from build123d import *

# Parameters (mm, degrees)
SALIENTE_EXTRUIR1_DEPTH    = 4.91
VACIADO1_T                 = -1.95
CROQUIS3_R                 = 2
SALIENTE_EXTRUIR3_DEPTH    = 2.96
CORTAR_EXTRUIR1_DEPTH      = 68.872038609
CORTAR_EXTRUIR1_DEPTH_BACK = 2.96
CROQUIS4_R                 = 1


with BuildPart() as part:
    # Croquis1 → Saliente-Extruir1 (new body)
    with BuildSketch(Plane.XY):
        Polygon((-54.055, -12.97), (-54.055, -40.75), (54.055, -40.75), (54.055, -12.97), (48.055, -12.97), (48.055, 12.97), (54.055, 12.97), (54.055, 40.75), (-54.055, 40.75), (-54.055, 12.97), (-48.055, 12.97), (-48.055, -12.97), align=None)
    extrude(amount=SALIENTE_EXTRUIR1_DEPTH)

    # Vaciado1
    vaciado1_openings = [part.faces().sort_by_distance(p)[0] for p in [
        (0, 0, 4.91),
    ]]
    offset(amount=VACIADO1_T, openings=vaciado1_openings, kind=Kind.INTERSECTION)

    # Croquis3 → Saliente-Extruir3 (add)
    with BuildSketch(Plane.XY):
        with Locations((-47.72, 30.01)):
            Circle(CROQUIS3_R)
        with Locations(Location((47.72, 30.01, 0), (0, 0, 180))):
            Circle(CROQUIS3_R)
        with Locations((47.72, -30.01)):
            Circle(CROQUIS3_R)
        with Locations(Location((-47.72, -30.01, 0), (0, 0, 180))):
            Circle(CROQUIS3_R)
    extrude(amount=SALIENTE_EXTRUIR3_DEPTH)

    # Croquis4 → Cortar-Extruir1 (cut, two sides: drawn at the far end of the back side and taken through both)
    with BuildSketch(Plane.XY.offset(-CORTAR_EXTRUIR1_DEPTH_BACK)):
        with Locations((-47.72, 30.01)):
            Circle(CROQUIS4_R)
        with Locations(Location((47.72, 30.01, 0), (0, 0, 180))):
            Circle(CROQUIS4_R)
        with Locations((47.72, -30.01)):
            Circle(CROQUIS4_R)
        with Locations(Location((-47.72, -30.01, 0), (0, 0, 180))):
            Circle(CROQUIS4_R)
    extrude(amount=CORTAR_EXTRUIR1_DEPTH + CORTAR_EXTRUIR1_DEPTH_BACK, mode=Mode.SUBTRACT)


solid = part.part
CAD build for the part. Positions are in the model's coordinates, mm. A direction names the side the tool comes from. Give positions to 0.01 mm unless a question says otherwise; leave off trailing zeros. Loops run counter-clockwise (first coordinate to the right, second up) from the corner with the lowest first, then second, coordinate; pieces in that order, holes last. Notation, with made-up numbers: M 22,86.25 L 41,86.25 A9 cw 41,99.25 Z; hole C 68,-18.5 d5. An arc over 180 degrees is marked long. Answer in a Markdown table with one row per item. Add a question column.
Item 1: Probe probe 1 along Y at (x, z) = (-47.72, 1.75); probe 2 along Y at (x, z) = (32, 3.75); probe 3 along X at (y, z) = (-24, 3.6) (3 decimals). List the from-to ranges inside material, lowest first.
Item 2: Tool access for faces 5 (the face through (-54.055, -27, 2)), 6 (the face through (51, -12.97, 2)), 7 (the face through (-45.873, 29.244, 2.448)), 8 (the face through (-48.055, 0, 2)): list every direction of +Z, -Z, +X, -X, +Y, -Y with a clear straight run to the whole face (end or side of a thin tool).
Item 3: Mould opens along Y. For faces 1 (the face through (49.567, -30.776, 2.448)), 2 (the face through (-1, -40.75, 2)), 3 (the face through (-54.055, 27, 2)), 4 (the face through (52.105, -27, 3)) say: +Y half, -Y half, draft (parallel to the pull), parting line (faces both ways), or undercut.
Item 4: Band-saw the part on B-B on x = 30.5. Give the cut face in (y, z), then the cut area to 3 significant figures.
Item 5: Drop flat-ended pins along their axis: P1, Ø1.5, axis at y = -4.5, z = 4, coming from the -X side (3 decimals); P2, Ø3, axis at x = 12.5, y = 22, coming from the +Z side; P3, Ø1.2, axis at x = -47.72, y = -30.01, coming from the +Z side; P4, Ø2, axis at x = 48.5, y = -30, coming from the +Z side. Give the stop position or say it passes through.
Item 6: Band-saw the part on A-A on y = 3.5. Give the cut face in (x, z) (3 decimals), then the cut area to 3 significant figures.
Reply:
| question | item | result |
|---|---|---|
| 1 | probe 1 | y = -40.75 to -31.01, -29.01 to 29.01, 31.01 to 40.75 |
| 1 | probe 2 | y = -40.75 to -38.8, 38.8 to 40.75 |
| 1 | probe 3 | x = -54.055 to -52.105, 52.105 to 54.055 |
| 2 | face 5 | +Z, -Z, -X, +Y, -Y |
| 2 | face 6 | +Z, -Z, +X |
| 2 | face 7 | +Z |
| 2 | face 8 | +Z, -Z, -X |
| 3 | face 1 | undercut |
| 3 | face 2 | -Y half |
| 3 | face 3 | draft |
| 3 | face 4 | undercut |
| 4 | outline | M -40.75,0 L 40.75,0 L 40.75,4.91 L 38.8,4.91 L 38.8,1.95 L -38.8,1.95 L -38.8,4.91 L -40.75,4.91 Z |
| 4 | area | 170 mm^2 |
| 5 | P1 | stops at x = -48.055 |
| 5 | P2 | stops at z = 1.95 |
| 5 | P3 | passes through |
| 5 | P4 | stops at z = 2.96 |
| 6 | outline | M -48.055,0 L 48.055,0 L 48.055,4.91 L 46.105,4.91 L 46.105,1.95 L -46.105,1.95 L -46.105,4.91 L -48.055,4.91 Z |
| 6 | area | 199 mm^2 |
